```python
from build123d import *

# Parameters (mm, degrees)
BOSS_EXTRUDE1_DEPTH = 3
SKETCH2_R           = 2.95
SKETCH2_R_2         = 9.95
BOSS_EXTRUDE2_DEPTH = 22
BOSS_EXTRUDE3_DEPTH = 3


with BuildPart() as part:
    # Sketch1 → Boss-Extrude1 (new body)
    with BuildSketch(Plane.XY):
        with BuildLine():
            Line((-7, 15), (75, 15))
            ThreePointArc((75, 15), (78.535533906, 13.535533906), (80, 10))
            Line((80, 10), (80, -10))
            ThreePointArc((80, -10), (78.535533906, -13.535533906), (75, -15))
            Line((75, -15), (-7, -15))
            ThreePointArc((-7, -15), (-10.535533906, -13.535533906), (-12, -10))
            Line((-12, -10), (-12, 10))
            ThreePointArc((-12, 10), (-10.535533906, 13.535533906), (-7, 15))
        make_face()
    extrude(amount=BOSS_EXTRUDE1_DEPTH)

    # Sketch2 → Boss-Extrude2 (add)
    with BuildSketch(Plane.XY.offset(3)):
        with Locations(Location((0, 0, 0), (0, 0, 180))):
            Circle(SKETCH2_R)
        with Locations(Location((60, 0, 0), (0, 0, 180))):
            Circle(SKETCH2_R_2)
    extrude(amount=BOSS_EXTRUDE2_DEPTH)

    # Sketch3 → Boss-Extrude3 (add)
    with BuildSketch(Plane.XY.offset(25)):
        with BuildLine():
            Line((75, 15), (-7, 15))
            ThreePointArc((-7, 15), (-10.535533906, 13.535533906), (-12, 10))
            Line((-12, 10), (-12, -10))
            ThreePointArc((-12, -10), (-10.535533906, -13.535533906), (-7, -15))
            Line((-7, -15), (75, -15))
            ThreePointArc((75, -15), (78.535533906, -13.535533906), (80, -10))
            Line((80, -10), (80, 10))
            ThreePointArc((80, 10), (78.535533906, 13.535533906), (75, 15))
        make_face()
    extrude(amount=BOSS_EXTRUDE3_DEPTH)


solid = part.part
```
Check sheet for the modelled part. Datum: model origin and axes. Units: mm. A direction names the side the tool comes from. Give positions to 0.01 mm unless a question says otherwise; leave off trailing zeros. Write each loop counter-clockwise with the first axis right and the second up, starting at its lowest first coordinate (ties: lowest second). Pieces come first, ordered by that corner, then holes. Notation, with made-up numbers: (-10, 3) -> (19, 3) arc R6 cw to (19, 12) -> close; hole circle Ø5 at (60.25, -28). An arc over 180 degrees is marked (long way). Use CSV: the item, a comma, the result in double quotes. Start each with the question number.
Q1. Cross-section at A-A on x = 46.5. Enter the section's corners in (y, z).
Q2. Tool access check on faces 1 (the flat face through (-12, 0, 1)), 2 (the cylindrical face through (69.94, -0.44, 13.85)). Record the directions out of +Z, -Z, +X, -X, +Y, -Y that give a thin tool (end or side, any length) a straight path to the whole face; none if there is none.
Q3. Cross-section at B-B on y = 13. Enter the section's corners in (x, z), and give its area (3 significant figures).
Q4. Release check for a two-part mould opening along X. For faces 3 (the cylindrical face through (-11, 13, 1)), 4 (the flat face through (80, 0, 1)), 5 (the cylindrical face through (2.947, -0.13, 13.846)) record: +X half, -X half, draft (parallel to the pull), parting line (faces both ways), or undercut.
Q5. Cross-section at C-C on z = 10.75. Enter the section's corners in (x, y), and give its area (3 significant figures).
Q6. Cross-section at D-D on y = 0. Enter the section's corners in (x, z).
Q7. Scan lines: line 1 along Z through (x, y) = (32, 13.25); line 2 along X through (y, z) = (-1, 23.25); line 3 along X through (y, z) = (-0.75, 7). Record each from-to range of solid material in increasing order.
Q8. Depth check by flat-ended pin: P1, Ø4, axis at x = 61.5, y = -11.5, coming from the -Z side; P2, Ø4, axis at y = 8, z = 9.5, coming from the +X side; P3, Ø4, axis at y = -9.5, z = 22, coming from the -X side; P4, Ø6, axis at x = -2.5, z = 12, coming from the -Y side. Enter the tip coordinate at first touch or a pass-through.
Working result:
1,outline,"(-15, 0) -> (15, 0) -> (15, 3) -> (-15, 3) -> close; (-15, 25) -> (15, 25) -> (15, 28) -> (-15, 28) -> close"
2,face 1,"+Z, -Z, -X, +Y, -Y"
2,face 2,"none"
3,outline,"(-11, 0) -> (79, 0) -> (79, 3) -> (-11, 3) -> close; (-11, 25) -> (79, 25) -> (79, 28) -> (-11, 28) -> close"
3,area,"540 mm^2"
4,face 3,"-X half"
4,face 4,"+X half"
4,face 5,"undercut"
5,outline,"circle Ø5.9 at (0, 0); circle Ø19.9 at (60, 0)"
5,area,"338 mm^2"
6,outline,"(-12, 0) -> (80, 0) -> (80, 3) -> (69.95, 3) -> (69.95, 25) -> (80, 25) -> (80, 28) -> (-12, 28) -> (-12, 25) -> (-2.95, 25) -> (-2.95, 3) -> (-12, 3) -> close; hole (2.95, 3) -> (50.05, 3) -> (50.05, 25) -> (2.95, 25) -> close"
7,line 1,"z = 0 to 3, 25 to 28"
7,line 2,"x = -2.78 to 2.78, 50.1 to 69.9"
7,line 3,"x = -2.85 to 2.85, 50.08 to 69.92"
8,P1,"stops at z = 0"
8,P2,"stops at x = 67.94"
8,P3,"stops at x = 53.46"
8,P4,"stops at y = -2.95"
